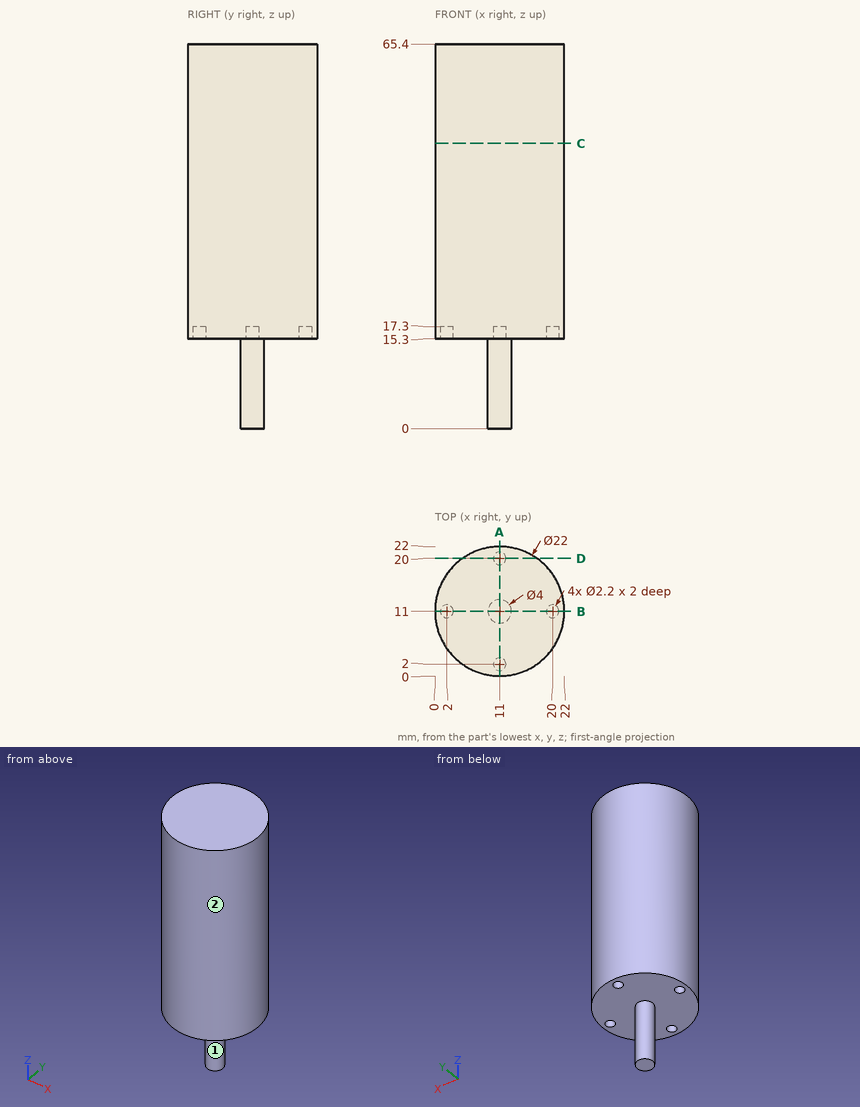
For this review, use the dimensioned drawing (mm, ordinates from the lowest corner) and the shaded views. A direction names the side the tool comes from. Give positions to 0.01 mm unless a question says otherwise; leave off trailing zeros. Write each loop counter-clockwise with the first axis right and the second up, starting at its lowest first coordinate (ties: lowest second). Pieces come first, ordered by that corner, then holes. Notation, with made-up numbers: M 83.25,89.5 L 91.25,89.5 A11 cw 91.25,108.5 Z; hole C 39,14 d9. An arc over 180 degrees is marked long. Answer as a JSON object with one key per item and string values. Group by question number.
1) We need section D-D (y = 20). Give the boundary of the cut face in (x, z).
2) For line 1 along Y through (x, z) = (11, 16.95); line 2 along Z through (x, y) = (6.75, 2), list the stretches that pass through material, from the lowest coordinate up.
3) Tool access review of the marked faces 1 and 2: name each direction out of +Z, -Z, +X, -X, +Y, -Y from which nothing blocks a thin tool from reaching the whole face with its end or side.
4) We need section A-A (x = 11). Give the boundary of the cut face in (y, z), and give its area (3 significant figures).
5) Clearance check with flat-ended pins moving along their axes: pin 1 Ø10 at (x, z) = (17, 28) entering from +Y; pin 2 Ø0.7 at (x, y) = (10.5, 20) entering from -Z; pin 3 Ø1.8 at (x, y) = (2.5, 10.5) entering from -Z. State where each tip first meets the part, or that it passes through.
6) We need section C-C (z = 48.5). Give the boundary of the cut face in (x, y), and give its area (3 significant figures).
Answer key:
{
 "1": {"outline": "M 4.68,15.3 L 9.9,15.3 L 9.9,17.3 L 12.1,17.3 L 12.1,15.3 L 17.32,15.3 L 17.32,65.4 L 4.68,65.4 Z"},
 "2": {"line 1": "y = 0 to 0.9, 3.1 to 18.9, 21.1 to 22", "line 2": "z = 15.3 to 65.4"},
 "3": {"face 1": "-Z", "face 2": "+Z, -Z"},
 "4": {"outline": "M 0,15.3 L 0.9,15.3 L 0.9,17.3 L 3.1,17.3 L 3.1,15.3 L 9,15.3 L 9,0 L 13,0 L 13,15.3 L 18.9,15.3 L 18.9,17.3 L 21.1,17.3 L 21.1,15.3 L 22,15.3 L 22,65.4 L 0,65.4 Z", "area": "1,150 mm²"},
 "5": {"pin 1": "stops at y = 21.95", "pin 2": "stops at z = 17.3", "pin 3": "stops at z = 15.3"},
 "6": {"outline": "C 11,11 d22", "area": "380 mm²"}
}
